For this review, take the finished solid that the model builds, in its own axes (mm). A direction names the side the tool comes from. Give positions to 0.01 mm unless a question says otherwise; leave off trailing zeros. Order: outer loops, then holes, each group sorted by start corner. A loop starts at its lowest first (then second) coordinate and runs counter-clockwise, first axis right, second up. Notation, with made-up numbers: M -30,75 L -22,75 A17 cw -22,91 Z; hole C 20.25,-29 d8. An arc over 180 degrees is marked long. Use CSV: the item, a comma, the result in double quotes. Start each with the question number.
(1) Consider section A-A (x = 12.5). Write out the cut boundary in (y, z), and give its area (3 significant figures).
(2) Consider section D-D (z = 215). Write out the cut boundary in (x, y).
(3) Consider section C-C (z = 370). Write out the cut boundary in (x, y).
(4) Draft analysis for pull direction Z (two halves, no side actions). For faces 1 (the face through (1.014, -15.154, 396.451)), 2 (the face through (0, -15, 207)), 3 (the face through (24.9, -28.3, 0)), state which applies: pulls with the +Z half, pulls with the -Z half, needs draft (parallel to the pull), parting line crosses it, or undercut.
(5) Clearance check with flat-ended pins moving along their axes: P1, Ø1, axis at x = 27.5, y = -0.5, coming from the -Z side; P2, Ø12, axis at x = 17, z = 249, coming from the +Y side. State where each tip first meets the part, or that it passes through.
(6) Wall thickness on L1, parallel to X at y = -28.8, z = 15; L2, parallel to Z at x = 0.6, y = -17; L3, parallel to X at y = -15.5, z = 305.5: over which ranges is each line inside the solid? List them lowest first. Write a range as from..to.
(7) Consider section B-B (y = -5.75). Write out the cut boundary in (x, z), and give its area (3 significant figures).
(8) Tool access review of faces 4 (the face through (41.466, -28.986, 14.479)), 5 (the face through (25, -2, 248)): name each direction out of +Z, -Z, +X, -X, +Y, -Y from which nothing blocks a thin tool from reaching the whole face with its end or side.
```python
from build123d import *

# Parameters (mm, degrees)
SKETCH1_W           = 50
SKETCH1_H           = 30
SKETCH1_W_2         = 46
SKETCH1_H_2         = 26
BOSS_EXTRUDE1_DEPTH = 420
SKETCH7_R           = 4
CUT_EXTRUDE2_DEPTH  = 424.89149555
SKETCH8_R           = 4
CUT_EXTRUDE3_DEPTH  = 425.028300942
CUT_EXTRUDE4_REACH  = 426.028
SKETCH9_W           = 46
SKETCH9_H           = 80


with BuildPart() as part:
    # Sketch1 → Boss-Extrude1 (new body)
    with BuildSketch(Plane.XY):
        with Locations((25, -15)):
            Rectangle(SKETCH1_W, SKETCH1_H)
        with Locations((25, -15)):
            Rectangle(SKETCH1_W_2, SKETCH1_H_2, mode=Mode.SUBTRACT)
    extrude(amount=BOSS_EXTRUDE1_DEPTH)

    # Sketch7 → Cut-Extrude2 (cut, through all)
    with BuildSketch(Plane(origin=(0, -28, 0), x_dir=(1, 0, 0), z_dir=(0, 1, 0))):
        with Locations(Location((37.5, -45, 0), (0, 0, 270))):
            Circle(SKETCH7_R)
        with Locations(Location((12.5, -45, 0), (0, 0, 270))):
            Circle(SKETCH7_R)
        with Locations(Location((12.5, -15, 0), (0, 0, 270))):
            Circle(SKETCH7_R)
        with Locations(Location((37.5, -15, 0), (0, 0, 270))):
            Circle(SKETCH7_R)
    extrude(amount=-CUT_EXTRUDE2_DEPTH, mode=Mode.SUBTRACT)

    # Sketch8 → Cut-Extrude3 (cut, through all)
    with BuildSketch(Plane(origin=(50, 0, 0), x_dir=(0, 0, -1), z_dir=(1, 0, 0))):
        with Locations(Location((-400, -17, 0), (0, 0, 90))):
            Circle(SKETCH8_R)
        with Locations(Location((-370, -17, 0), (0, 0, 90))):
            Circle(SKETCH8_R)
    extrude(amount=-CUT_EXTRUDE3_DEPTH, mode=Mode.SUBTRACT)

    # Sketch9 → Cut-Extrude4 (cut, up to next)
    with BuildSketch(Plane(origin=(0, 0, 0), x_dir=(1, 0, 0), z_dir=(0, 1, 0)), mode=Mode.PRIVATE) as cut_extrude4_sk1:
        with Locations((25, -40)):
            Rectangle(SKETCH9_W, SKETCH9_H)
    cut_extrude4_tool1 = extrude(cut_extrude4_sk1.sketch, amount=-CUT_EXTRUDE4_REACH, mode=Mode.PRIVATE) & part.part
    add(cut_extrude4_tool1.solids().sort_by_distance((25, 0, 40))[0], mode=Mode.SUBTRACT)


solid = part.part
```
Check result:
1,outline,"M -30,0 L -28,0 L -28,11 L -30,11 Z; M -30,19 L -28,19 L -28,41 L -30,41 Z; M -30,49 L -28,49 L -28,420 L -30,420 Z; M -2,80 L 0,80 L 0,420 L -2,420 Z"
1,area,"1,490 mm^2"
2,outline,"M 0,-30 L 50,-30 L 50,0 L 0,0 Z; hole M 2,-28 L 48,-28 L 48,-2 L 2,-2 Z"
3,outline,"M 0,-30 L 50,-30 L 50,-21 L 48,-21 L 48,-28 L 2,-28 L 2,-21 L 0,-21 Z; M 0,-13 L 2,-13 L 2,-2 L 48,-2 L 48,-13 L 50,-13 L 50,0 L 0,0 Z"
4,face 1,"undercut"
4,face 2,"needs draft"
4,face 3,"pulls with the -Z half"
5,P1,"stops at z = 80"
5,P2,"stops at y = 0"
6,L1,"x = 0..8.5, 16.5..33.5, 41.5..50"
6,L2,"z = 0..366, 374..396, 404..420"
6,L3,"x = 0..2, 48..50"
7,outline,"M 0,0 L 2,0 L 2,420 L 0,420 Z; M 48,0 L 50,0 L 50,420 L 48,420 Z"
7,area,"1,680 mm^2"
8,face 4,"+Y, -Y"
8,face 5,"+Z, -Z"
